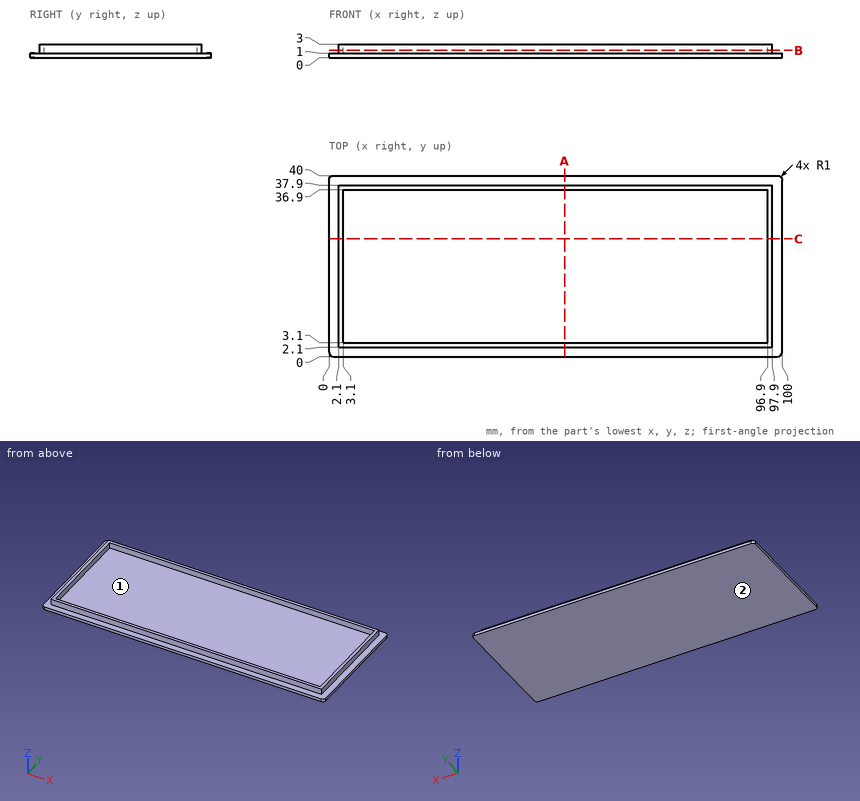
The figure shows three views and two pictorial views of one solid part (mm, origin at its lowest corner). Answer the questions. A direction names the side the tool comes from. Round coordinates to 2 decimals unless told otherwise and drop trailing zeros. Loops run counter-clockwise (first coordinate to the right, second up) from the corner with the lowest first, then second, coordinate; pieces in that order, holes last. Notation, with made-up numbers: M 68.25,64 L 78.25,64 A32 cw 78.25,91 Z; hole C -30.5,-7 d6. An arc over 180 degrees is marked long. Write each question's results on one line, items separated by ' | '. Start each with the question number.
1) Which of the six approach directions +Z, -Z, +X, -X, +Y, -Y give full straight-line access (tool end or side, diameter ignored) to the marked faces 1 and 2?
2) Each of these flat-tipped pins is pushed along its axis until it touches: pin 1 (1.6 mm diameter, centred on x = 41, z = 2.5, fed in from -Y); pin 2 (1.6 mm diameter, centred on x = 66.5, z = 2, fed in from +Y); pin 3 (12 mm diameter, centred on x = 85.5, y = 28.5, fed in from +Z). Where does it stop, or does it pass through?
3) Find section A-A on x = 52. Write down the section's boundary in (y, z).
4) Find section B-B on z = 1.6. Write down the section's boundary in (x, y).
5) Straight lines are drawn through the part: probe 1 along Y at (x, z) = (66, 1.55); probe 2 along X at (y, z) = (31.5, 1.7); probe 3 along Z at (x, y) = (7.5, 27). For each, find the intervals that lie inside material, in ascending order.
6) Find section C-C on y = 26. Write down the section's boundary in (x, z).
Final values:
1) face 1: +Z | face 2: -Z, +X, -X, +Y, -Y
2) pin 1: y = 2.1 | pin 2: y = 37.9 | pin 3: z = 1
3) outline: M 0,0 L 40,0 L 40,1 L 37.9,1 L 37.9,3 L 36.9,3 L 36.9,1 L 3.1,1 L 3.1,3 L 2.1,3 L 2.1,1 L 0,1 Z
4) outline: M 2.1,2.1 L 97.9,2.1 L 97.9,37.9 L 2.1,37.9 Z; hole M 3.1,3.1 L 96.9,3.1 L 96.9,36.9 L 3.1,36.9 Z
5) probe 1: 2.1 to 3.1, 36.9 to 37.9 | probe 2: 2.1 to 3.1, 96.9 to 97.9 | probe 3: 0 to 1
6) outline: M 0,0 L 100,0 L 100,1 L 97.9,1 L 97.9,3 L 96.9,3 L 96.9,1 L 3.1,1 L 3.1,3 L 2.1,3 L 2.1,1 L 0,1 Z
